For this review, take the finished solid that the model builds, in its own axes (mm). A direction names the side the tool comes from. Round coordinates to 2 decimals unless told otherwise and drop trailing zeros. Write each loop counter-clockwise with the first axis right and the second up, starting at its lowest first coordinate (ties: lowest second). Pieces come first, ordered by that corner, then holes. Notation, with made-up numbers: (6.25, 71.25) -> (13.25, 71.25) arc R31 cw to (13.25, 101.25) -> close; hole circle Ø11 at (-19, -11.75). An arc over 180 degrees is marked (long way). Write each question's results on one line, items separated by ' | '. Start each with the question number.
Item 1: Add section A-A (z = 15). State the section outline as (x, y) points (3 decimals), plus the area to 3 significant figures.
Item 2: Add section C-C (y = 31). State the section outline as (x, z) points, plus the area to 3 significant figures.
Item 3: To check wall thickness, follow line 1 along Y through (x, z) = (0, 8.75); line 2 along X through (y, z) = (46, 55); line 3 along Z through (x, y) = (40.25, 82.55). State the ranges of each line that lie inside material, in increasing order.
Item 4: The part is to be moulded in two halves that separate along Y. For faces 1 (the cylindrical face through (82.556, 19.329, 6.261)), 2 (the flat face through (0, 120.65, 12)), 3 (the flat face through (107.95, 56, 7)), say which applies: +Y half, -Y half, draft (parallel to the pull), parting line (faces both ways), or undercut.
Item 5: Add section D-D (z = 69.85). State the section outline as (x, y) points (3 decimals).
Item 6: Clearance check with flat-ended pins moving along their axes: pin 1 (24 mm diameter, centred on x = 83, y = 32, fed in from +Z); pin 2 (10 mm diameter, centred on x = 88.9, y = 95.25, fed in from -Z); pin 3 (5 mm diameter, centred on y = 96.5, z = 30.5, fed in from +X); pin 4 (3 mm diameter, centred on y = 87.5, z = 29, fed in from -X). State where each tip first meets the part, or that it passes through.
Item 7: Add section B-B (x = 42.5). State the section outline as (y, z) points, plus the area to 3 significant figures.
Item 8: Tool access review of faces 4 (the flat face through (76, 24, 12.7)), 5 (the flat face through (39.11, 34.47, 72.54)), 6 (the flat face through (52, 52, 76.2)), 7 (the flat face through (76, 89, 12.7)), 8 (the flat face through (32.669, 75, 49)): name each direction out of +Z, -Z, +X, -X, +Y, -Y from which nothing blocks a thin tool from reaching the whole face with its end or side.
from build123d import *

# Parameters (mm, degrees)
F0_R     = 6.35
F1_DEPTH = 12.7
F0_W     = 69.85
F0_H     = 120.65
F0_R_2   = 7.9375
F0_W_2   = 12.7
F2_DEPTH = 107.95
F0_W_3   = 62.5805897668
F0_H_2   = 9.525
F3_DEPTH = 76.2
F5_DEPTH = 25.4
F6_R     = 19.05
F7_DEPTH = 159.6704102332


with BuildPart() as f1:
    # F0 (on Top) → F1 (new body)
    with BuildSketch(Plane.XY):
        Polygon((91.5022938823, 120.65), (45.3694102332, 120.65), (45.3694102332, 57.15), (107.95, 57.15), (107.95, 101.6), align=None)
        with Locations((88.9, 95.25)):
            Circle(F0_R, mode=Mode.SUBTRACT)
    extrude(amount=F1_DEPTH)



with BuildPart() as f1b:
    # F0 (on Top) → F1, piece 2 (new body)
    with BuildSketch(Plane.XY):
        Polygon((45.3694102332, 47.625), (45.3694102332, 0), (91.5022938823, 0), (107.95, 11.4125879677), (107.95, 47.625), align=None)
        with Locations((88.9, 19.05)):
            Circle(F0_R, mode=Mode.SUBTRACT)
    extrude(amount=F1_DEPTH)


with BuildPart() as f1c:
    # F0 (on Top) → F1, piece 3 (new body)
    with BuildSketch(Plane.XY):
        with Locations((-2.2555897668, 60.325)):
            Rectangle(F0_W, F0_H)
        with Locations((0, 25.4)):
            Circle(F0_R_2, mode=Mode.SUBTRACT)
        with Locations((0, 101.6)):
            Circle(F0_R_2, mode=Mode.SUBTRACT)
    extrude(amount=F1_DEPTH)


with BuildPart() as f1d:
    # F0 (on Top) → F1, piece 4 (new body)
    with BuildSketch(Plane.XY):
        Polygon((-114.3, 0), (-91.3736136669, 0), (-49.8805897668, 0), (-49.8805897668, 120.65), (-114.3, 38.1), align=None)
        with Locations((-95.25, 12.7)):
            Circle(F0_R, mode=Mode.SUBTRACT)
    extrude(amount=F1_DEPTH)


with BuildPart() as f1_1:
    add(f1.part)

    add(f1b.part)  # F2 merges F1b

    add(f1c.part)  # F2 merges F1c

    add(f1d.part)  # F2 merges F1d
    # F0 (on Top) → F2 (join)
    with BuildSketch(Plane.XY):
        with Locations((-43.5305897668, 60.325)):
            Rectangle(F0_W_2, F0_H)
        Polygon((32.6694102332, 120.65), (32.6694102332, 0), (45.3694102332, 0), (45.3694102332, 47.625), (45.3694102332, 57.15), (45.3694102332, 120.65), align=None)
    extrude(amount=F2_DEPTH)

    # F0 (on Top) → F3 (join)
    with BuildSketch(Plane.XY):
        with Locations((76.6597051166, 52.3875)):
            Rectangle(F0_W_3, F0_H_2)
    extrude(amount=F3_DEPTH)

    # F4 (on face) → F5 (cut)
    with BuildSketch(Plane(origin=(0, 57.15, 0), x_dir=(-1, 0, 0), z_dir=(0, 1, 0))):
        Polygon((-107.95, 76.2), (-107.95, 25.4), (-58.0694102332, 76.2), align=None)
    extrude(amount=-F5_DEPTH, mode=Mode.SUBTRACT)

    # F6 (on face) → F7 (cut, through all)
    with BuildSketch(Plane.YZ.offset(45.3694102332)):
        Polygon((0, 107.95), (0, 38.1), (69.9122603316, 107.95), align=None)
        Polygon((120.65, 107.95), (108.0122603316, 107.95), (120.65, 93.6955257524), align=None)
        with Locations((82.55, 69.85)):
            Circle(F6_R)
    extrude(amount=-F7_DEPTH, mode=Mode.SUBTRACT)


solid = f1_1.part
Responses:
1) outline: (-49.881, 0) -> (-37.181, 0) -> (-37.181, 120.65) -> (-49.881, 120.65) -> close; (32.669, 0) -> (45.369, 0) -> (45.369, 47.625) -> (107.95, 47.625) -> (107.95, 57.15) -> (45.369, 57.15) -> (45.369, 120.65) -> (32.669, 120.65) -> close | area: 3,660 mm^2
2) outline: (-114.3, 0) -> (-5.63, 0) -> (-5.63, 12.7) -> (-37.18, 12.7) -> (-37.18, 69.07) -> (-49.88, 69.07) -> (-49.88, 12.7) -> (-114.3, 12.7) -> close; (5.63, 0) -> (107.95, 0) -> (107.95, 12.7) -> (45.37, 12.7) -> (45.37, 69.07) -> (32.67, 69.07) -> (32.67, 12.7) -> (5.63, 12.7) -> close | area: 4,110 mm^2
3) line 1: y = 0 to 17.46, 33.34 to 93.66, 109.54 to 120.65 | line 2: x = -49.88 to -37.18, 32.67 to 45.37 | line 3: z = 0 to 50.8, 88.9 to 107.95
4) face 1: undercut | face 2: +Y half | face 3: draft
5) outline: (-49.881, 31.778) -> (-37.181, 31.778) -> (-37.181, 63.5) -> (-49.881, 63.5) -> close; (-49.881, 101.6) -> (-37.181, 101.6) -> (-37.181, 120.65) -> (-49.881, 120.65) -> close; (32.669, 31.778) -> (45.369, 31.778) -> (45.369, 47.625) -> (64.304, 47.625) -> (64.304, 57.15) -> (45.369, 57.15) -> (45.369, 63.5) -> (32.669, 63.5) -> close; (32.669, 101.6) -> (45.369, 101.6) -> (45.369, 120.65) -> (32.669, 120.65) -> close
6) pin 1: stops at z = 12.7 | pin 2: passes through | pin 3: stops at x = 45.37 | pin 4: stops at x = -49.88
7) outline: (0, 0) -> (120.65, 0) -> (120.65, 93.7) -> (108.01, 107.95) -> (69.91, 107.95) -> (0, 38.1) -> close; hole circle Ø38.1 at (82.55, 69.85) | area: 9,350 mm^2
8) face 4: +Z, +X, -Y | face 5: +Z, +X, -X, -Y | face 6: +Z, +X, +Y, -Y | face 7: +Z, +X, +Y | face 8: +Z, +Y, -Y
